For this review, take the finished solid that the model builds, in its own axes (mm). A direction names the side the tool comes from. Round coordinates to 2 decimals unless told otherwise and drop trailing zeros. Loops run counter-clockwise (first coordinate to the right, second up) from the corner with the lowest first, then second, coordinate; pieces in that order, holes last.
1) Take a section at A-A (x = 1.5). State the section outline as (y, z) points, then the cut area to 3 significant figures.
2) Tool access review of faces 1 (the flat face through (1, 0, -5)), 2 (the flat face through (4, 1.9, -5)): name each direction out of +Z, -Z, +X, -X, +Y, -Y from which nothing blocks a thin tool from reaching the whole face with its end or side.
3) Take a section at D-D (y = 1). State the section outline as (x, z) points.
4) Take a section at B-B (y = 3.5). State the section outline as (x, z) points.
5) Take a section at C-C (z = -5.5). State the section outline as (x, y) points, then the cut area to 3 significant figures.
6) Insertion check: pin 1 (0.7 mm diameter, centred on y = 3.5, z = -5.5, fed in from -X); pin 2 (1 mm diameter, centred on x = 5.5, z = -1.5, fed in from -Y). Each pin has a flat end and moves straight along its axis. Give the tip position at first contact, or say it passes through.
7) Wall thickness on L1, parallel to X at y = 3.5, z = -6.25; L2, parallel to Y at x = 6.5, z = -6; L3, parallel to X at y = 0.8, z = -1: over which ranges is each line inside the solid? List them lowest first.
8) Mouldability with a two-part tool opening along X and no side actions: class faces 3 (the flat face through (7, 0, -5)), 4 (the flat face through (1.32, 1, -5)), 5 (the flat face through (0, 2, -5)) as pulls with the +X half, pulls with the -X half, needs draft (parallel to the pull), parting line crosses it, or undercut.
```python
from build123d import *

# Parameters (mm, degrees)
SKETCH1_W           = 7.74
SKETCH1_H           = 4.92
BOSS_EXTRUDE1_DEPTH = 10
SKETCH2_W           = 5.1
SKETCH2_H           = 1.9
CUT_EXTRUDE1_DEPTH  = 11
SKETCH3_W           = 0.32
SKETCH3_H           = 0.64
SKETCH3_W_2         = 0.64
CUT_EXTRUDE2_DEPTH  = 11


with BuildPart() as part:
    # Sketch1 → Boss-Extrude1 (new body)
    with BuildSketch(Plane.XY):
        with Locations((3.87, 2.46)):
            Rectangle(SKETCH1_W, SKETCH1_H)
    extrude(amount=-BOSS_EXTRUDE1_DEPTH)

    # Sketch2 → Cut-Extrude1 (cut, through all)
    with BuildSketch(Plane.XY):
        with Locations((3.87, 0.95)):
            Rectangle(SKETCH2_W, SKETCH2_H)
    extrude(amount=-CUT_EXTRUDE1_DEPTH, mode=Mode.SUBTRACT)

    # Sketch3 → Cut-Extrude2 (cut, through all)
    with BuildSketch(Plane.XY):
        with Locations((3.71, 3.6)):
            Rectangle(SKETCH3_W, SKETCH3_H)
        with Locations((1.34, 3.6)):
            Rectangle(SKETCH3_W_2, SKETCH3_H)
    cut_extrude2 = extrude(amount=-CUT_EXTRUDE2_DEPTH, mode=Mode.SUBTRACT)

    # Mirror1: Cut-Extrude2 across plane
    add(cut_extrude2.mirror(Plane.ZY.offset(-3.87)), mode=Mode.SUBTRACT)


solid = part.part
```
Response:
1. outline: (1.9, -10) - (3.28, -10) - (3.28, 0) - (1.9, 0) - close; (3.92, -10) - (4.92, -10) - (4.92, 0) - (3.92, 0) - close
1. area: 23.8 mm2
2. face 1: +Z, -Z, +X, -X, -Y
2. face 2: +Z, -Z, -Y
3. outline: (0, -10) - (1.32, -10) - (1.32, 0) - (0, 0) - close; (6.42, -10) - (7.74, -10) - (7.74, 0) - (6.42, 0) - close
4. outline: (0, -10) - (1.02, -10) - (1.02, 0) - (0, 0) - close; (1.66, -10) - (3.55, -10) - (3.55, 0) - (1.66, 0) - close; (4.19, -10) - (6.08, -10) - (6.08, 0) - (4.19, 0) - close; (6.72, -10) - (7.74, -10) - (7.74, 0) - (6.72, 0) - close
5. outline: (0, 0) - (1.32, 0) - (1.32, 1.9) - (6.42, 1.9) - (6.42, 0) - (7.74, 0) - (7.74, 4.92) - (0, 4.92) - close; hole (1.02, 3.28) - (1.66, 3.28) - (1.66, 3.92) - (1.02, 3.92) - close; hole (3.55, 3.28) - (4.19, 3.28) - (4.19, 3.92) - (3.55, 3.92) - close; hole (6.08, 3.28) - (6.72, 3.28) - (6.72, 3.92) - (6.08, 3.92) - close
5. area: 27.2 mm2
6. pin 1: stops at x = 0
6. pin 2: stops at y = 1.9
7. L1: x = 0 to 1.02, 1.66 to 3.55, 4.19 to 6.08, 6.72 to 7.74
7. L2: y = 0 to 3.28, 3.92 to 4.92
7. L3: x = 0 to 1.32, 6.42 to 7.74
8. face 3: needs draft
8. face 4: undercut
8. face 5: pulls with the -X half
